Part model, mm, in its own coordinate system. A direction names the side the tool comes from. Round coordinates to 2 decimals unless told otherwise and drop trailing zeros. Write each loop counter-clockwise with the first axis right and the second up, starting at its lowest first coordinate (ties: lowest second). Pieces come first, ordered by that corner, then holes. Notation, with made-up numbers: M 45.25,-32.75 L 49.25,-32.75 A9 cw 49.25,-24.75 Z; hole C 25,-30 d10. An arc over 180 degrees is marked long. One line per question, with ' | ' between items. Start each with the question number.
1) Tool access for faces 5 (the face through (3.22, -27.83, -18.51)), 6 (the face through (3, -6.35, -2)): list every direction of +Z, -Z, +X, -X, +Y, -Y with a clear straight run to the whole face (end or side of a thin tool).
2) Mould opens along Y. For faces 1 (the face through (3.22, -26.91, -55.17)), 2 (the face through (6.35, -7, -20)), 3 (the face through (3, -6.35, 35)), 4 (the face through (3.219, 27.082, -17.215)) say: pulls with the +Y half, pulls with the -Y half, needs draft (parallel to the pull), parting line crosses it, or undercut.
3) Saw through at A-A (z = -57.15). List the corners of the cut face in (x, y).
4) Saw through at B-B (y = 25.4). List the corners of the cut face in (x, z).
5) Saw through at C-C (z = 44.45). List the corners of the cut face in (x, y).
6) Drop a flat-ended pin along its axis: pin 1 Ø1.9 at (x, y) = (3, 16.5) entering from +Z. Give the stop position or say it passes through.
7) Saw through at D-D (x = 2.25). List the corners of the cut face in (y, z) (3 decimals).
8) Wall check: probe 1 along Y at (x, z) = (5, -57.15); probe 2 along Y at (x, z) = (1.5, 44.45); probe 3 along Y at (x, z) = (4.5, -20). Give the ranges that are in metal, low to high. Write a range as [from, to].
```python
from build123d import *

# Parameters (mm, degrees)
BOSS_EXTRUDE1_DEPTH            = 6.35
F_9_0_196_DIAMETER_HOLE1_D     = 4.9784
F_9_0_196_DIAMETER_HOLE1_DEPTH = 70.104
F_9_0_196_DIAMETER_HOLE1_TIP   = 1.495662253
F_9_0_196_DIAMETER_HOLE2_D     = 4.9784
F_9_0_196_DIAMETER_HOLE2_DEPTH = 70.104
F_9_0_196_DIAMETER_HOLE2_TIP   = 1.495662253
Z_0_413_DIAMETER_HOLE1_D       = 10.4902
Z_0_413_DIAMETER_HOLE1_DEPTH   = 70.104
Z_0_413_DIAMETER_HOLE1_TIP     = 3.151574033


with BuildPart() as part:
    # Sketch1 → Boss-Extrude1 (new body)
    with BuildSketch(Plane(origin=(0, 0, 0), x_dir=(0, 0, -1), z_dir=(1, 0, 0))):
        Polygon((-50.8, -6.35), (12.7, -6.35), (12.7, 31.75), (63.5, 31.75), (63.5, -31.75), (-50.8, -31.75), align=None)
    extrude(amount=BOSS_EXTRUDE1_DEPTH)

    # #9 (0.196) Diameter Hole1
    with Locations(Plane.ZY):
        with Locations((44.45, -22.225), (-6.35, -22.225)):
            Hole(F_9_0_196_DIAMETER_HOLE1_D / 2, depth=F_9_0_196_DIAMETER_HOLE1_DEPTH)
            with Locations((0, 0, -(F_9_0_196_DIAMETER_HOLE1_DEPTH + F_9_0_196_DIAMETER_HOLE1_TIP / 2))):  # 118° drill point
                Cone(0, F_9_0_196_DIAMETER_HOLE1_D / 2, F_9_0_196_DIAMETER_HOLE1_TIP, mode=Mode.SUBTRACT)

    # #9 (0.196) Diameter Hole2
    with Locations(Plane.ZY):
        with Locations((-57.15, -25.4), (-19.05, -25.4), (-19.05, 25.4), (-57.15, 25.4)):
            Hole(F_9_0_196_DIAMETER_HOLE2_D / 2, depth=F_9_0_196_DIAMETER_HOLE2_DEPTH)
            with Locations((0, 0, -(F_9_0_196_DIAMETER_HOLE2_DEPTH + F_9_0_196_DIAMETER_HOLE2_TIP / 2))):  # 118° drill point
                Cone(0, F_9_0_196_DIAMETER_HOLE2_D / 2, F_9_0_196_DIAMETER_HOLE2_TIP, mode=Mode.SUBTRACT)

    # Z (0.413) Diameter Hole1
    with Locations(Plane.ZY):
        with Locations((12.7, -6.35)):
            Hole(Z_0_413_DIAMETER_HOLE1_D / 2, depth=Z_0_413_DIAMETER_HOLE1_DEPTH)
            with Locations((0, 0, -(Z_0_413_DIAMETER_HOLE1_DEPTH + Z_0_413_DIAMETER_HOLE1_TIP / 2))):  # 118° drill point
                Cone(0, Z_0_413_DIAMETER_HOLE1_D / 2, Z_0_413_DIAMETER_HOLE1_TIP, mode=Mode.SUBTRACT)


solid = part.part
```
Answer key:
1) face 5: +X, -X | face 6: +Z, +X, -X, +Y
2) face 1: undercut | face 2: needs draft | face 3: pulls with the +Y half | face 4: undercut
3) outline: M 0,-31.75 L 6.35,-31.75 L 6.35,-27.89 L 0,-27.89 Z; M 0,-22.91 L 6.35,-22.91 L 6.35,22.91 L 0,22.91 Z; M 0,27.89 L 6.35,27.89 L 6.35,31.75 L 0,31.75 Z
4) outline: M 0,-63.5 L 6.35,-63.5 L 6.35,-59.64 L 0,-59.64 Z; M 0,-54.66 L 6.35,-54.66 L 6.35,-21.54 L 0,-21.54 Z; M 0,-16.56 L 6.35,-16.56 L 6.35,-12.7 L 0,-12.7 Z
5) outline: M 0,-31.75 L 6.35,-31.75 L 6.35,-24.71 L 0,-24.71 Z; M 0,-19.74 L 6.35,-19.74 L 6.35,-6.35 L 0,-6.35 Z
6) pin 1: stops at z = -12.7
7) outline: M -31.75,-63.5 L 31.75,-63.5 L 31.75,-12.7 L -6.35,-12.7 L -6.35,7.455 A5.245 cw -6.35,17.945 L -6.35,50.8 L -31.75,50.8 Z; hole C -25.4,-57.15 d4.978; hole C -25.4,-19.05 d4.978; hole C -22.225,-6.35 d4.978; hole C -22.225,44.45 d4.978; hole C 25.4,-57.15 d4.978; hole C 25.4,-19.05 d4.978
8) probe 1: y = [-31.75, -27.89], [-22.91, 22.91], [27.89, 31.75] | probe 2: y = [-31.75, -24.71], [-19.74, -6.35] | probe 3: y = [-31.75, -27.7], [-23.1, 23.1], [27.7, 31.75]
